Autodesk Inventor part; units mm, degrees
ref_plane "YZ Plane" through (0, 0, 0) normal (1, 0, 0) x (0, 1, 0)
ref_plane "XZ Plane" through (0, 0, 0) normal (0, 1, 0) x (-1, 0, 0)
ref_plane "XY Plane" through (0, 0, 0) normal (0, 0, 1) x (1, 0, 0)
sketch "Schizzo1" plane through (0, 0, 0) normal (0, 0, 1) x (1, 0, 0)
  circle A0 centre (0, 0) radius 9
  dimension "d0" = 18
extrude "Estrusione1" add sketch "Schizzo1" along normal blind 77
thread "Filettatura1"
chamfer "Smusso1" distance 1 angle 45 1 edges at (-9, 0, 77)
sketch "Schizzo3" plane through (0, 0, 0) normal (0, 0, -1) x (-1, 0, 0)
  circle A0 centre (0, 0) radius 1
  dimension "d8" = 2
sketch "Schizzo4" plane through (0, 0, 0) normal (1, 0, 0) x (0, 1, 0)
  line L0 (-9, 0) -> (9, 0)
  line L1 (3.6716, 0) -> (6.4362, -4.8477) construction
  line L2 (6.4362, -4.8477) -> (2.6524, -12.3111) construction
  line L3 (2.6524, -12.3111) -> (0, -13.9912) construction
  line L4 (0, -13.9912) -> (4.2654, -31.599) construction
  spline S0 degree 4 poles (3.6716, 0) (6.4362, -4.8477) (2.6524, -12.3111) (0, -13.9912) (4.2654, -31.599) knots 1 1 1 1 1 2 2 2 2 2
  point P0 (0, 0)
sweep "Sweep1" add profiles "Schizzo3" path "Schizzo4" path curves S0
properties part number "Modello sensore ultrasuoni" material "Plastica ABS"
Part model, mm, in its own coordinate system. Round coordinates to 2 decimals unless told otherwise and drop trailing zeros. Write each loop counter-clockwise with the first axis right and the second up, starting at its lowest first coordinate (ties: lowest second). Pieces come first, ordered by that corner, then holes.
Item 1: Drop flat-ended pins along their axis: pin 1 Ø1.5 at (x, z) = (3, -0.5) entering from +Y; pin 2 Ø1 at (x, z) = (-1, 40) entering from +Y; pin 3 Ø1 at (x, z) = (-0.5, -5) entering from +Y; pin 4 Ø6 at (y, z) = (-2.5, 26) entering from +X. Give the stop position or say it passes through.
Results:
pin 1: stops at y = 8.66
pin 2: stops at y = 8.99
pin 3: stops at y = 2.25
pin 4: stops at x = 9
Item 2: Probe L1, parallel to Y at x = -0.25, z = 2; L2, parallel to Z at x = -4, y = 5.75; L3, parallel to X at y = -5.75, z = 31.5. List the from-to ranges inside material, lowest first.
Results:
L1: y = -9 to 9
L2: z = 0 to 77
L3: x = -6.92 to 6.92
Item 3: Cut at A-A, the plane z = 29.5. Give the cut face in (x, y).
Results:
outline: circle Ø18 at (0, 0)
